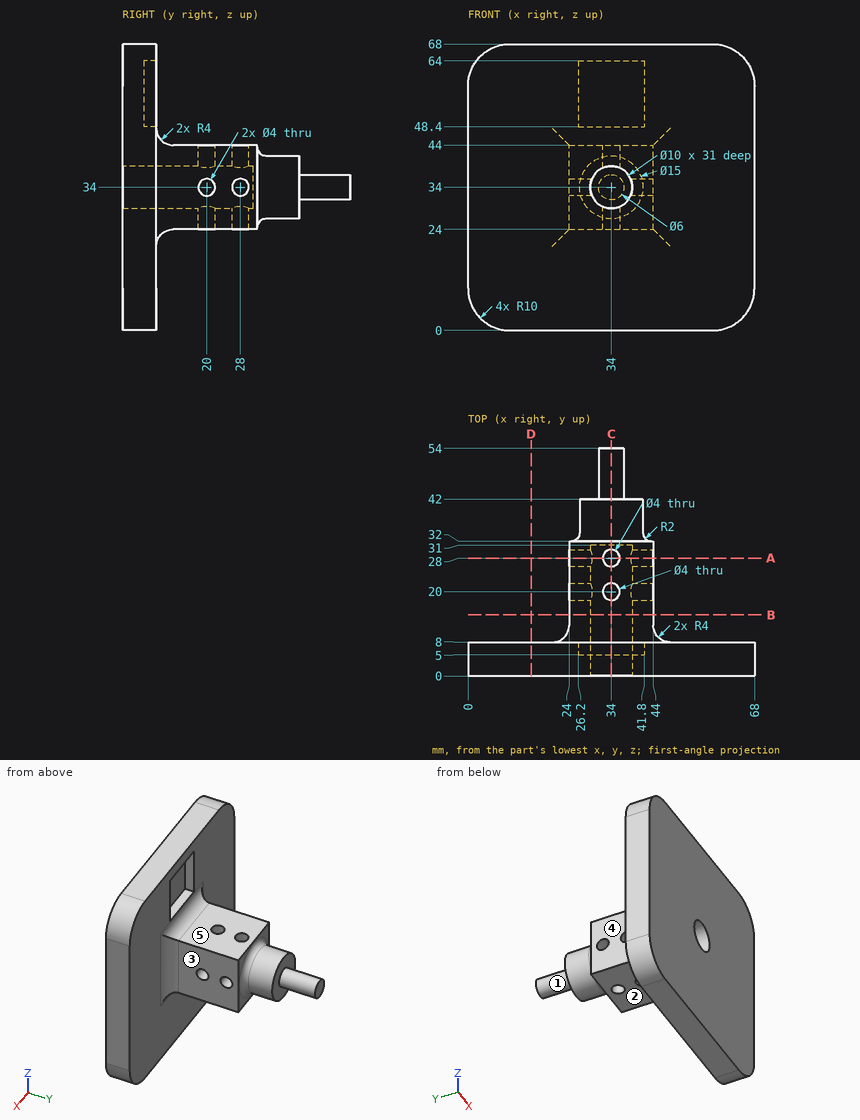
Check sheet for the drawn part. Datum: minimum x, y, z corner. Units: mm. A direction names the side the tool comes from. Round coordinates to 2 decimals unless told otherwise and drop trailing zeros. Order: outer loops, then holes, each group sorted by start corner. A loop starts at its lowest first (then second) coordinate and runs counter-clockwise, first axis right, second up.
1. Go/stop test with flat-tipped pins: P1, Ø16, axis at y = 26.5, z = 35.5, coming from the +X side; P2, Ø4, axis at x = 44, y = 45, coming from the +Z side; P3, Ø11, axis at x = 34.5, z = 34, coming from the -Y side; P4, Ø6, axis at x = 36.5, y = 26, coming from the +Z side. Record where each tip stops, or that it passes through.
Final values:
P1: stops at x = 44
P2: passes through
P3: stops at y = 0
P4: stops at z = 44
2. Access from +Z, -Z, +X, -X, +Y, -Y to the whole of each face (thin tool, end or side, straight path). Record for the marked faces 1, 2, 3, 4 and 5.
Final values:
face 1: +Y
face 2: -Z, +X, -X, +Y
face 3: +Z, -Z, +X, +Y
face 4: +Z, -Z, -X, +Y
face 5: +Z, +X, -X, +Y
3. Section check B-B on y = 14.5. Record the cut outline in (x, z).
Final values:
outline: (24, 24) - (44, 24) - (44, 44) - (24, 44) - close; hole circle Ø10 at (34, 34)
4. Section check A-A on y = 28. Record the cut outline in (x, z).
Final values:
outline: (24, 24) - (32, 24) - (32, 29.42) arc R5 cw to (29.42, 32) - (24, 32) - close; (24, 36) - (29.42, 36) arc R5 cw to (32, 38.58) - (32, 44) - (24, 44) - close; (36, 24) - (44, 24) - (44, 32) - (38.58, 32) arc R5 cw to (36, 29.42) - close; (36, 38.58) arc R5 cw to (38.58, 36) - (44, 36) - (44, 44) - (36, 44) - close
5. Section check D-D on x = 15. Record the cut outline in (y, z).
Final values:
outline: (0, 0) - (8, 0) - (8, 68) - (0, 68) - close
6. Section check C-C on x = 34. State how many separate pieces and enclosed holes the cut face has, then the cut area to 3 significant figures.
Final values:
separate pieces: 5
enclosed holes: 0
area: 818 mm2
7. Thickness scan on L1, parallel to Y at x = 25, z = 34; L2, parallel to Y at x = 31.5, z = 60; L3, parallel to X at y = 31.5, z = 36. Record the ranges inside material, lowest first.
Final values:
L1: y = 0 to 18, 22 to 26, 30 to 32.06
L2: y = 0 to 5
L3: x = 24 to 44
